Read the model definition and answer for the solid it produces. Units are mm, in the model's axes. A direction names the side the tool comes from. Give positions to 0.01 mm unless a question says otherwise; leave off trailing zeros. Loops run counter-clockwise (first coordinate to the right, second up) from the corner with the lowest first, then second, coordinate; pieces in that order, holes last. Notation, with made-up numbers: (27, -28) - (50, -28) arc R15 ccw to (50, -22) - close; hole circle Ø11 at (64.25, 2.5). An arc over 180 degrees is marked (long way). Put each result on its own line as item: value. Start each with the question number.
1. A cutting plane is placed at B-B, the plane z = 14. Determine the outline of the cut face in (x, y), plus the area to 3 significant figures.
2. A cutting plane is placed at D-D, the plane z = 0. Determine the outline of the cut face in (x, y).
3. A cutting plane is placed at A-A, the plane x = -14. Determine the outline of the cut face in (y, z).
4. Consider L1, parallel to Z at x = 14, y = 0.5; L2, parallel to Y at x = -2, z = -6. Determine where each line is inside the solid, lowest interval first. Write a range as from..to.
5. For a pull along Z with two mould halves and no side action, classify faces 1 (the cylindrical face through (-13.762, 0.789, 15.074)), 2 (the flat face through (5.4, 5.1, -5.4)), 3 (the cylindrical face through (6.834, 15.62, 1.517)) as released by +Z, released by -Z, zero draft, split by the parting line, or undercut.
6. A cutting plane is placed at C-C, the plane x = 6. Determine the outline of the cut face in (y, z).
7. Given pin 1 Ø0.8 at (y, z) = (-1, -12) entering from -X; pin 2 Ø1.4 at (x, y) = (0.5, -1.5) entering from -Z; pin 3 Ø10 at (x, z) = (0.5, -1) entering from -Y, each flat-ended and moving along its own axis, determine where each tip first touches the part or whether it passes through.
8. For faces 4 (the cylindrical face through (-11.003, 3.326, 0.042)), 5 (the flat face through (0, -1, -10.38)), 6 (the flat face through (5, -1, -13)), determine the directions among +Z, -Z, +X, -X, +Y, -Y from which every point of the face is accessible in a straight line to the end or side of a thin tool.
```python
from build123d import *

# Parameters (mm, degrees)
SKETCH_1_W         = 32
SKETCH_1_H         = 32
EXTRUDE_1_DEPTH    = 1.6
HOLE_WIZARD_M2_1_D = 2.2
SKETCH_4_W         = 10
SKETCH_4_H         = 4.7
EXTRUDE_2_DEPTH    = 1.7
EXTRUDE_4_DEPTH    = 3.5
SKETCH_7_R         = 7
EXTRUDE_5_DEPTH    = 5
SKETCH_8_R         = 5.5
EXTRUDE_6_DEPTH    = 3.4
SKETCH_9_R         = 7
EXTRUDE_7_DEPTH    = 4.3


with BuildPart() as part:
    # 草图1 → 凸台-拉伸1 (new body)
    with BuildSketch(Plane(origin=(0, 0, 0), x_dir=(1, 0, 0), z_dir=(0, 1, 0))):
        Rectangle(SKETCH_1_W, SKETCH_1_H)
    extrude(amount=EXTRUDE_1_DEPTH)

    # M2 间隙孔1 (through all)
    with Locations(Plane(origin=(0, 1.6, 0), x_dir=(1, 0, 0), z_dir=(0, 1, 0))):
        with Locations((-14, 14), (14, 14), (14, -14), (-14, -14)):
            Hole(HOLE_WIZARD_M2_1_D / 2)

    # 草图4 → 凸台-拉伸2 (add)
    with BuildSketch(Plane(origin=(0, 0, 0), x_dir=(1, 0, 0), z_dir=(0, 1, 0))):
        with Locations((0, 12.73)):
            Rectangle(SKETCH_4_W, SKETCH_4_H)
    extrude(amount=-EXTRUDE_2_DEPTH)

    # 草图6 → 凸台-拉伸4 (add)
    with BuildSketch(Plane(origin=(0, 1.6, 0), x_dir=(1, 0, 0), z_dir=(0, 1, 0))):
        with BuildLine():
            Line((-6.5, 6.5), (6.5, 6.5))
            Line((6.5, 6.5), (6.5, 2))
            Line((6.5, 2), (9, 2))
            ThreePointArc((9, 2), (11, 0), (9, -2))
            Line((9, -2), (6.5, -2))
            Line((6.5, -2), (6.5, -6.5))
            Line((6.5, -6.5), (-6.5, -6.5))
            Line((-6.5, -6.5), (-6.5, -2))
            Line((-6.5, -2), (-9.119024186, -2))
            ThreePointArc((-9.119024186, -2), (-11.003538559, 0), (-9.119024186, 2))
            Line((-9.119024186, 2), (-6.5, 2))
            Line((-6.5, 2), (-6.5, 6.5))
        make_face()
    extrude(amount=EXTRUDE_4_DEPTH)

    # 草图7 → 凸台-拉伸5 (add)
    with BuildSketch(Plane(origin=(0, 5.1, 0), x_dir=(1, 0, 0), z_dir=(0, 1, 0))):
        with Locations(Location((-0.001769279, 0, 0), (0, 0, 68.213210702))):
            Circle(SKETCH_7_R)
    extrude(amount=EXTRUDE_5_DEPTH)

    # 草图8 → 凸台-拉伸6 (add)
    with BuildSketch(Plane(origin=(0, 10.1, 0), x_dir=(1, 0, 0), z_dir=(0, 1, 0))):
        with Locations(Location((0, 0, 0), (0, 0, 270))):
            Circle(SKETCH_8_R)
    extrude(amount=EXTRUDE_6_DEPTH)

    # 草图9 → 凸台-拉伸7 (add)
    with BuildSketch(Plane(origin=(0, 13.5, 0), x_dir=(1, 0, 0), z_dir=(0, 1, 0))):
        with Locations(Location((0, 0, 0), (0, 0, 90))):
            Circle(SKETCH_9_R)
    extrude(amount=EXTRUDE_7_DEPTH)


solid = part.part
```
Return value:
1. outline: (-16, 0) - (-15.1, 0) - (-15.1, 1.6) - (-16, 1.6) - close; (-12.9, 0) - (12.9, 0) - (12.9, 1.6) - (-12.9, 1.6) - close; (15.1, 0) - (16, 0) - (16, 1.6) - (15.1, 1.6) - close
1. area: 44.2 mm2
2. outline: (-16, 0) - (16, 0) - (16, 1.6) - (11, 1.6) - (11, 5.1) - (7, 5.1) - (7, 10.1) - (5.5, 10.1) - (5.5, 13.5) - (7, 13.5) - (7, 17.8) - (-7, 17.8) - (-7, 13.5) - (-5.5, 13.5) - (-5.5, 10.1) - (-7, 10.1) - (-7, 5.1) - (-11, 5.1) - (-11, 1.6) - (-16, 1.6) - close
3. outline: (0, -16) - (1.6, -16) - (1.6, -15.1) - (0, -15.1) - close; (0, -12.9) - (1.6, -12.9) - (1.6, 12.9) - (0, 12.9) - close; (0, 15.1) - (1.6, 15.1) - (1.6, 16) - (0, 16) - close
4. L1: z = -16..-15.1, -12.9..12.9, 15.1..16
4. L2: y = 0..10.1, 13.5..17.8
5. face 1: undercut
5. face 2: zero draft
5. face 3: split by the parting line
6. outline: (0, -16) - (1.6, -16) - (1.6, -6.5) - (5.1, -6.5) - (5.1, -3.6) - (10.1, -3.6) - (10.1, 3.6) - (5.1, 3.6) - (5.1, 6.5) - (1.6, 6.5) - (1.6, 16) - (0, 16) - close; (13.5, -3.61) - (17.8, -3.61) - (17.8, 3.61) - (13.5, 3.61) - close
7. pin 1: stops at x = -5
7. pin 2: stops at z = -15.08
7. pin 3: stops at y = 0
8. face 4: -X, +Y
8. face 5: +Z, +X, -X, -Y
8. face 6: +Z, -Z, +X, -Y
